from build123d import *

# Parameters (mm, degrees)
JACKET_START        = -32
SKETCH_1_R          = 56
SKETCH_1_R_2        = 54
JACKET_DEPTH        = 52
REAR_FLANGE_START   = -32
SKETCH_2_R          = 61
SKETCH_2_R_2        = 54
REAR_FLANGE_DEPTH   = 3
FRONT_FLANGE_START  = 18
SKETCH_3_R          = 61
SKETCH_3_R_2        = 54
FRONT_FLANGE_DEPTH  = 2
SKETCH_4_R          = 1.65
THROUGH_HOLES_DEPTH = 100


with BuildPart() as part:
    # Эскиз1 → Jacket (new body)
    with BuildSketch(Plane.XY.offset(JACKET_START)):
        with Locations(Location((0, 0, 0), (0, 0, 180))):
            Circle(SKETCH_1_R)
        with Locations(Location((0, 0, 0), (0, 0, 180))):
            Circle(SKETCH_1_R_2, mode=Mode.SUBTRACT)
    extrude(amount=JACKET_DEPTH)

    # Эскиз2 → Rear_flange (add)
    with BuildSketch(Plane.XY.offset(REAR_FLANGE_START)):
        Circle(SKETCH_2_R)
        with Locations(Location((0, 0, 0), (0, 0, 180))):
            Circle(SKETCH_2_R_2, mode=Mode.SUBTRACT)
    extrude(amount=REAR_FLANGE_DEPTH)

    # Эскиз3 → Front_flange (add)
    with BuildSketch(Plane.XY.offset(FRONT_FLANGE_START)):
        Circle(SKETCH_3_R)
        with Locations(Location((0, 0, 0), (0, 0, 180))):
            Circle(SKETCH_3_R_2, mode=Mode.SUBTRACT)
    extrude(amount=FRONT_FLANGE_DEPTH)

    # Эскиз4 → Through_holes (cut, symmetric)
    with BuildSketch(Plane.XY):
        with Locations((58, 0)):
            Circle(SKETCH_4_R)
        with Locations((29, 50.229473419)):
            Circle(SKETCH_4_R)
        with Locations((-29, 50.229473419)):
            Circle(SKETCH_4_R)
        with Locations((-58, 0)):
            Circle(SKETCH_4_R)
        with Locations((-29, -50.229473419)):
            Circle(SKETCH_4_R)
        with Locations((29, -50.229473419)):
            Circle(SKETCH_4_R)
    extrude(amount=THROUGH_HOLES_DEPTH, both=True, mode=Mode.SUBTRACT)


solid = part.part
Design review of the part built by this model. Coordinates are the model's own, in mm. A direction names the side the tool comes from. Give positions to 0.01 mm unless a question says otherwise; leave off trailing zeros. Loops run counter-clockwise (first coordinate to the right, second up) from the corner with the lowest first, then second, coordinate; pieces in that order, holes last. Notation, with made-up numbers: (76, -15.5) - (132, -15.5) arc R11 ccw to (132, 4.5) - close; hole circle Ø8 at (-6, 73.25). An arc over 180 degrees is marked (long way). Write item = value, one per line.
1) Clearance check with flat-ended pins moving along their axes: pin 1 Ø2 at (x, z) = (31, -22) entering from +Y; pin 2 Ø5 at (y, z) = (-15.5, -17) entering from +X; pin 3 Ø3 at (x, z) = (20, -0.5) entering from +Y. State where each tip first meets the part, or that it passes through.
Result sheet:
pin_1 = 47.29
pin_2 = 54.47
pin_3 = 52.86
2) Take a section at B-B on y = 0. Count the separate pieces of the cut face and the enclosed holes in it, and give its area (3 significant figures).
Result sheet:
separate_pieces = 6
enclosed_holes = 0
area = 225 mm2
3) Tool access review of faces 1 (the face through (-51.73, 21.45, -5.83)), 2 (the face through (27.691, 49.225, -30.479)): name each direction out of +Z, -Z, +X, -X, +Y, -Y from which nothing blocks a thin tool from reaching the whole face with its end or side.
Result sheet:
face_1 = none
face_2 = +Z, -Z
4) Draft analysis for pull direction Y (two halves, no side actions). For faces 3 (the face through (-48.408, -37.118, -30.521)), 4 (the face through (26.8, -49.4, 18)), 5 (the face through (27.691, 49.225, 18.986)), state which applies: +Y half, -Y half, draft (parallel to the pull), parting line (faces both ways), or undercut.
Result sheet:
face_3 = parting line
face_4 = draft
face_5 = undercut
5) To check wall thickness, follow line 1 (Y direction, x = 29, z = -30); line 2 (Z direction, x = -55, y = 21.5); line 3 (Y direction, x = 23, z = 9). State the ranges of each line that lie inside material, in increasing order.
Result sheet:
line_1 = -53.67 to -51.88, -48.58 to -45.55, 45.55 to 48.58, 51.88 to 53.67
line_2 = -32 to -29, 18 to 20
line_3 = -51.06 to -48.86, 48.86 to 51.06
6) Take a section at C-C on y = -47. State the section outline as (x, z) points, and give its area (3 significant figures).
Result sheet:
outline = (-38.88, -32) - (-26.59, -32) - (-26.59, 20) - (-38.88, 20) - (-38.88, 18) - (-30.45, 18) - (-30.45, -29) - (-38.88, -29) - close; (26.59, -32) - (38.88, -32) - (38.88, -29) - (30.45, -29) - (30.45, 18) - (38.88, 18) - (38.88, 20) - (26.59, 20) - close
area = 486 mm2
7) Take a section at A-A on x = 0. State the section outline as (y, z) points.
Result sheet:
outline = (-61, -32) - (-54, -32) - (-54, 20) - (-61, 20) - (-61, 18) - (-56, 18) - (-56, -29) - (-61, -29) - close; (54, -32) - (61, -32) - (61, -29) - (56, -29) - (56, 18) - (61, 18) - (61, 20) - (54, 20) - close
